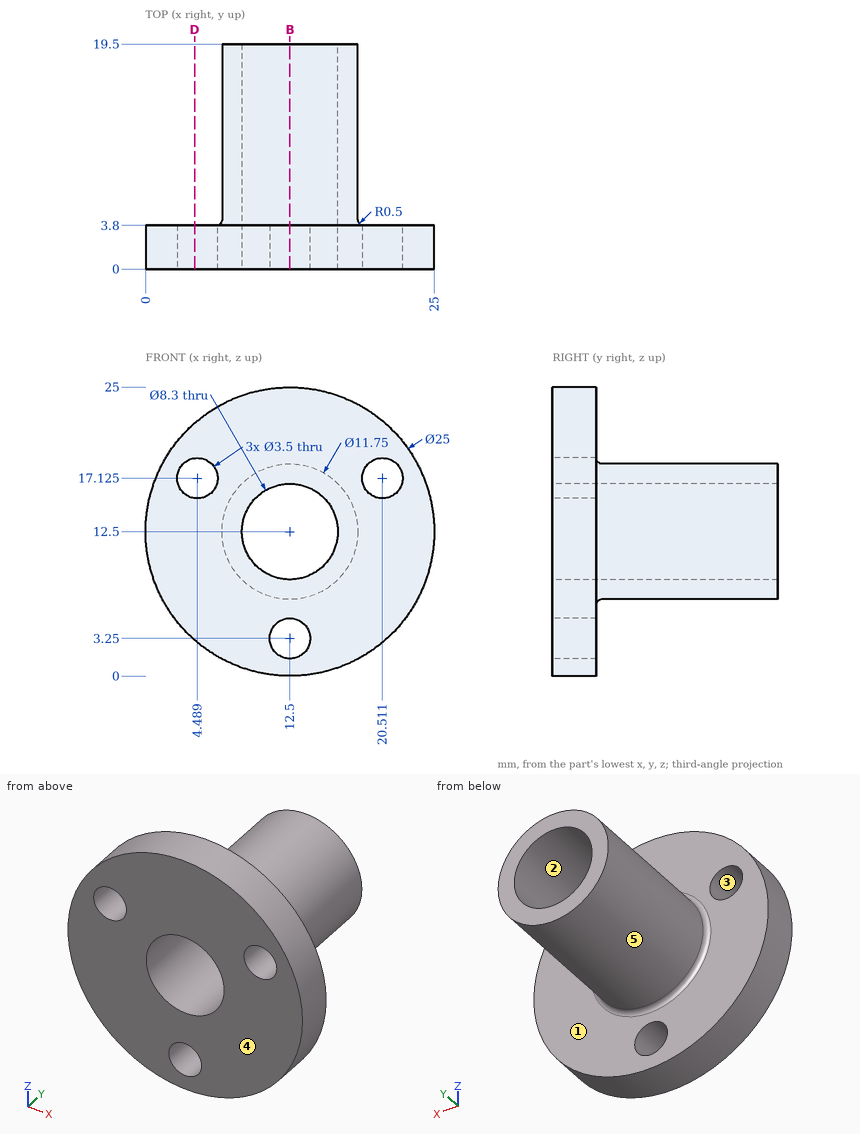
Input: dimensioned drawing with shaded views. Units: mm. Origin: part minimum x, y, z. A direction names the side the tool comes from. Coordinates: 2 decimals unless noted, no trailing zeros. Order: outer loops, then holes, each group sorted by start corner. A loop starts at its lowest first (then second) coordinate and runs counter-clockwise, first axis right, second up. Notation, with made-up numbers: M 53,3 L 59,3 A26 cw 59,19 Z; hole C -13,-14.5 d9. An arc over 180 degrees is marked long. Answer as CSV lines item,"result".
Q1. Section D-D on x = 4.25. Return the cut outline in (y, z).
Answers:
outline,"M 0,3.11 L 3.8,3.11 L 3.8,15.39 L 0,15.39 Z; M 0,18.86 L 3.8,18.86 L 3.8,21.89 L 0,21.89 Z"
Q2. Section B-B on x = 12.5. Count the separate pieces of the cut face and the enclosed holes in it, and give its area (3 significant figures).
Answers:
separate pieces,"3"
enclosed holes,"0"
area,"104 mm^2"
Q3. Draft query along Z for the marked faces 3, 4 and 5. Return one class per face: pulls with the +Z half, pulls with the -Z half, needs draft (parallel to the pull), parting line crosses it, or undercut.
Answers:
face 3,"undercut"
face 4,"needs draft"
face 5,"parting line crosses it"
Q4. Line query: probe 1 along Z at (x, y) = (12.5, 2.8); probe 2 along Z at (x, y) = (9.5, 7.75); probe 3 along Y at (x, z) = (18.75, 11.75). Output: solid intervals per line, ascending. Write a range as [from, to].
Answers:
probe 1,"z = [0, 1.5], [5, 8.35], [16.65, 25]"
probe 2,"z = [7.45, 9.63], [15.37, 17.55]"
probe 3,"y = [0, 3.81]"
Q5. First-contact query: P1, Ø1, axis at x = 15.5, z = 19.5, coming from the +Y side; P2, Ø4, axis at x = 21, y = 4, coming from the -Z side; P3, Ø10, axis at x = 20, y = 13.5, coming from the +Z side. Flat tips, straight axial feed; report the tip coordinate or a pass-through.
Answers:
P1,"stops at y = 3.8"
P2,"stops at z = 1.83"
P3,"stops at z = 17.82"
Q6. Set-up query: the marked faces 1 and 2. Return all of +Z, -Z, +X, -X, +Y, -Y with unobstructed straight access to the full face (end or side cutting, diameter ignored); none if empty.
Answers:
face 1,"+Y"
face 2,"+Y, -Y"
